Could you check a few things on this model? Use its own coordinates, in mm. A direction names the side the tool comes from. Coordinates: 2 decimals unless noted, no trailing zeros. Write each loop counter-clockwise with the first axis right and the second up, starting at its lowest first coordinate (ties: lowest second). Pieces come first, ordered by that corner, then holes. Notation, with made-up numbers: M 28,5 L 43,5 A8 cw 43,11 Z; hole C 49.5,2.25 d3. An arc over 180 degrees is marked long. Write item = value, one per line.
```python
from build123d import *

# Parameters (mm, degrees)
SKETCH_W = 1
SKETCH_H = 20


with BuildPart() as part:
    # AdditivePipe: sweep along a path in Sketch001
    with BuildLine(Plane.XY) as additivepipe_path:
        Line((0, 0), (-30, 0))
        ThreePointArc((-30, 0), (-35.748611, 7.718568), (-26.706875, 11.015509))
        Line((-26.706875, 11.015509), (-26.362344, 10.789294))
        ThreePointArc((-26.362344, 10.789294), (-19.361462, 12.345669), (-21.118073, 19.299011))
        Line((-21.118073, 19.299011), (-22.850124, 20.299011))
        ThreePointArc((-22.850124, 20.299011), (-25.103298, 26.180698), (-19.81394, 29.600306))
        ThreePointArc((-19.81394, 29.600306), (-17.013872, 30.113353), (-14.947628, 32.071474))
        Line((-14.947628, 32.071474), (5.052372, 66.71249))
    # Sketch → AdditivePipe (sweep)
    with BuildSketch(Plane.YZ):
        with Locations((0, 10)):
            Rectangle(SKETCH_W, SKETCH_H)
    sweep(path=additivepipe_path.line)


solid = part.part
```
Item 1: If we mould it in two halves opening along Y, with no side actions, what happens to faces 4 (the face through (-15, -0.5, 10)), 5 (the face through (-36.274, 7.699, 9.86)), 6 (the face through (-25.61, 26.24, 9.86))? For each: pulls with the +Y half, pulls with the -Y half, needs draft (parallel to the pull), parting line crosses it, or undercut.
Numbers:
face_4 = pulls with the -Y half
face_5 = parting line crosses it
face_6 = undercut
Item 2: Imagine slicing it at D-D (z = 12.75). Write out the boundary of the cut face in (x, y), and give its area (3 significant figures).
Numbers:
outline = M -30,-0.5 L 0,-0.5 L 0,0.5 L -30,0.5 A5.5 cw long -26.98,10.6 L -26.64,10.37 A5.5 ccw long -20.87,19.73 L -22.6,20.73 A4.5 cw -19.87,29.1 A5.5 ccw -14.51,31.82 L 5.49,66.46 L 4.62,66.96 L -15.38,32.32 A4.5 cw -19.76,30.1 A5.5 ccw -23.1,19.87 L -21.37,18.87 A4.5 cw long -26.09,11.21 L -26.43,11.43 A6.5 ccw long Z
area = 130 mm²
Item 3: If I drill on line 1 along Y through (x, z) = (-30, 14.5); line 2 along Y through (x, z) = (-21, 3.75); line 3 along Y through (x, z) = (-20.5, 4.5), over which ranges is the centre line in solid material (lowest first)?
Numbers:
line_1 = -0.5 to 0.5, 11.5 to 12.5
line_2 = -0.5 to 0.5, 10.13 to 11.31, 18.63 to 19.81, 29.08 to 30.09
line_3 = -0.5 to 0.5, 10.44 to 11.72, 18.21 to 19.5, 29.13 to 30.13
Item 4: I'm going to push flat-ended pins straight in: P1, Ø12, axis at x = -22.5, z = 3, coming from the +Y side; P2, Ø12, axis at x = -13.5, y = 22, coming from the -Z side; P3, Ø1.5, axis at y = 31.5, z = 17, coming from the -X side; P4, Ø6, axis at y = 9.5, z = 13, coming from the -X side. Where does each tip first touch, or does it pass through?
Numbers:
P1 = 31.03
P2 = through
P3 = -16.9
P4 = -36.48
Item 5: Imagine slicing it at B-B (x = -24). Write out the boundary of the cut face in (y, z), and give its area (3 significant figures).
Numbers:
outline = M -0.5,0 L 0.5,0 L 0.5,20 L -0.5,20 Z; M 9.48,0 L 10.49,0 L 10.49,20 L 9.48,20 Z; M 20.51,0 L 22,0 L 22,20 L 20.51,20 Z; M 27.26,0 L 28.74,0 L 28.74,20 L 27.26,20 Z
area = 99.3 mm²
Item 6: Imagine slicing it at A-A (x = -32.5). Write out the boundary of the cut face in (y, z).
Numbers:
outline = M 0,0 L 1.1,0 L 1.1,20 L 0,20 Z; M 10.9,0 L 12,0 L 12,20 L 10.9,20 Z
Item 7: Imagine slicing it at C-C (y = 6). Write out the boundary of the cut face in (x, z).
Numbers:
outline = M -36.5,0 L -35.5,0 L -35.5,20 L -36.5,20 Z
Item 8: For faces 1 (the face through (-22.246, 19.373, 10.14)), 2 (the face through (-4.375, 49.384, 9.86)), 3 (the face through (-5.241, 49.884, 10.14)), which set-ups out of +Z, -Z, +X, -X, +Y, -Y let a thin tool reach every point of the face, with its end or its side?
Numbers:
face_1 = +Z, -Z, -X
face_2 = +Z, -Z, +X
face_3 = +Z, -Z, -X, +Y
